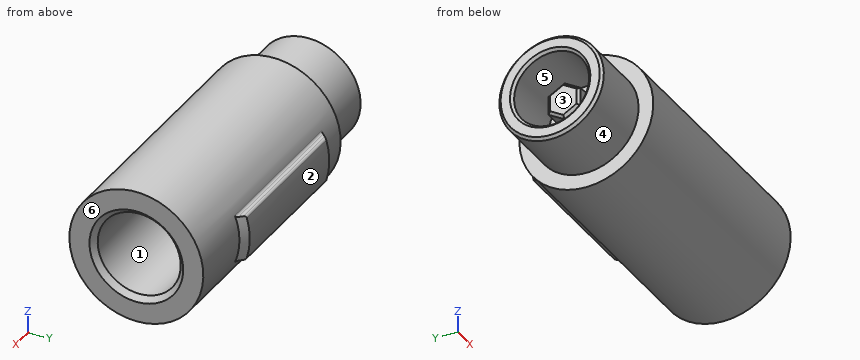
```python
from build123d import *

# Parameters (mm, degrees)
SKETCH_1_R          = 5
EXTRUDE_1_DEPTH     = 19
SKETCH_3_R          = 3.1
CUT_EXTRUDE_1_DEPTH = 17
EXTRUDE_2_DEPTH     = 12
SKETCH_8_R          = 3.9
EXTRUDE_4_DEPTH     = 5
SKETCH_9_R          = 2.8
CUT_EXTRUDE_2_DEPTH = 5
EXTRUDE_5_DEPTH     = 3.2
FILLET_1_R          = 0.2
CHAMFER_1_SIZE      = 0.5
CHAMFER_2_SIZE      = 0.4
CHAMFER_3_SIZE      = 0.2


with BuildPart() as part:
    # 草图1 → 凸台-拉伸1 (new body)
    with BuildSketch(Plane(origin=(0, 0, 0), x_dir=(0, 0, -1), z_dir=(1, 0, 0))):
        Circle(SKETCH_1_R)
    extrude(amount=EXTRUDE_1_DEPTH)

    # 草图3 → 切除-拉伸1 (cut)
    with BuildSketch(Plane(origin=(19, 0, 0), x_dir=(0, 0, -1), z_dir=(1, 0, 0))):
        Circle(SKETCH_3_R)
    extrude(amount=-CUT_EXTRUDE_1_DEPTH, mode=Mode.SUBTRACT)

    # 草图5 → 凸台-拉伸2 (add)
    with BuildSketch(Plane(origin=(2, 0, 0), x_dir=(0, 0, -1), z_dir=(1, 0, 0))):
        with BuildLine():
            Line((-1.688194302, 2.6), (1.688194302, 2.6))
            Line((1.688194302, 2.6), (1.688194302, 5.234500931))
            ThreePointArc((1.688194302, 5.234500931), (0, 5.5), (-1.688194302, 5.234500931))
            Line((-1.688194302, 5.234500931), (-1.688194302, 2.6))
        make_face()
    extrude(amount=EXTRUDE_2_DEPTH)

    # 草图8 → 凸台-拉伸4 (add)
    with BuildSketch(Plane.ZY):
        Circle(SKETCH_8_R)
    extrude(amount=EXTRUDE_4_DEPTH)

    # 草图9 → 切除-拉伸2 (cut)
    with BuildSketch(Plane.ZY.offset(5)):
        Circle(SKETCH_9_R)
    extrude(amount=-CUT_EXTRUDE_2_DEPTH, mode=Mode.SUBTRACT)

    # 草图10 → 凸台-拉伸5 (add)
    with BuildSketch(Plane.ZY):
        Polygon((0.692820323, 1.2), (-0.692820323, 1.2), (-1.385640646, 0), (-0.692820323, -1.2), (0.692820323, -1.2), (1.385640646, 0), align=None)
    extrude(amount=EXTRUDE_5_DEPTH)

    # 圆角1
    fillet_1_edges = [part.edges().sort_by_distance(p)[0] for p in [
        (8, 4.70637865, 1.688194302),
        (8, 5.234500931, 1.688194302),
        (8, 4.70637865, -1.688194302),
        (8, 5.234500931, -1.688194302),
    ]]
    fillet(fillet_1_edges, radius=FILLET_1_R)

    # 倒角1
    # the kernel refuses this chamfer: 0.5 mm, written as the material it takes off along each edge
    with BuildSketch(Plane(origin=(14, 0, 0), x_dir=(0, 0.8686030413593419, -0.4955085837211114), z_dir=(0, -0.4955085837211114, -0.8686030413593419))) as chamfer_1_piece_1:
        Polygon((5.5, -CHAMFER_1_SIZE), (5.5 - CHAMFER_1_SIZE, 0), (5.5, 0), align=None)
    revolve(axis=Axis((14, 0, 0), (1, 0, 0)), revolution_arc=59.40658503, mode=Mode.SUBTRACT)
    with BuildSketch(Plane(origin=(2, 0, 0), x_dir=(0, 0.8686030413593415, -0.4955085837211117), z_dir=(0, -0.4955085837211117, -0.8686030413593415))) as chamfer_1_piece_2:
        Polygon((5.5 - CHAMFER_1_SIZE, 0), (5.5, CHAMFER_1_SIZE), (5.5, 0), align=None)
    revolve(axis=Axis((2, 0, 0), (1, 0, 0)), revolution_arc=59.40658503, mode=Mode.SUBTRACT)
    with BuildSketch(Plane(origin=(14, 2.6, 2.974035796), x_dir=(0.027495876610585623, 0.9996219169112968, 0), z_dir=(0, 0, -1))) as chamfer_1_piece_3_section:
        Polygon((CHAMFER_1_SIZE * 0.999621916911, -CHAMFER_1_SIZE * 0.0274958766106), (-CHAMFER_1_SIZE * 0.0274958766106, -CHAMFER_1_SIZE * 0.999621916911), (0, 0), align=None)
    chamfer_1_piece_3 = extrude(amount=5.948071591, mode=Mode.PRIVATE)
    chamfer_1_piece_3 = chamfer_1_piece_3 & Plane(origin=(13.821912141, 0, 0), x_dir=(0, 0, -1), z_dir=(1, 0, 0)) * Cylinder(3.1, 14, mode=Mode.PRIVATE)
    add(chamfer_1_piece_3, mode=Mode.SUBTRACT)

    # 倒角2
    chamfer_2_edges = [part.edges().sort_by_distance(p)[0] for p in [
        (19, 0, 3.1),
    ]]
    chamfer(chamfer_2_edges, length=CHAMFER_2_SIZE)

    # 倒角3
    chamfer_3_edges = [part.edges().sort_by_distance(p)[0] for p in [
        (-5, 0, -3.9),
        (-5, 0, -2.8),
        (-3.2, 0.6, 1.039230485),
        (-3.2, 1.2, 0),
        (-3.2, 0.6, -1.039230485),
        (-3.2, -0.6, -1.039230485),
        (-3.2, -1.2, 0),
        (-3.2, -0.6, 1.039230485),
    ]]
    chamfer(chamfer_3_edges, length=CHAMFER_3_SIZE)


solid = part.part
```
Read the model definition and answer for the solid it produces. Units are mm, in the model's axes. Face numbers are marked on the shaded views. A direction names the side the tool comes from. Give positions to 0.01 mm unless a question says otherwise; leave off trailing zeros. Write each loop counter-clockwise with the first axis right and the second up, starting at its lowest first coordinate (ties: lowest second). Pieces come first, ordered by that corner, then holes. Notation, with made-up numbers: (-37, -33) - (3, -33) arc R19 ccw to (3, 2) - close; hole circle Ø11 at (53, 21.25). An arc over 180 degrees is marked (long way). Write item = value, one per line. Start each with the question number.
Item 1: Each of these flat-tipped pins is pushed along its axis until it touches: P1, Ø1, axis at x = 6.5, y = 2, coming from the +Z side; P2, Ø0.7, axis at x = -2, z = 0, coming from the +Y side; P3, Ø3, axis at y = 1, z = 0, coming from the -X side. Where does it stop, or does it pass through?
Item 2: Find the intervals of material crossed by probe 1 along Y at (x, z) = (-1.5, 0); probe 2 along Y at (x, z) = (13.25, 0); probe 3 along Y at (x, z) = (15.25, 0), in increasing order. Write a range as [from, to].
Item 3: Find section C-C (x = 10). Give the vertices of the cut face in (y, z), then the cut area to 3 significant figures.
Item 4: A tool of negligible diameter and unlimited length cuts with its end or side. For the marked faces 1, 2 and 3, from which of +Z, -Z, +X, -X, +Y, -Y can it reach the whole face along a straight path? Write none if from no direction.
Item 5: Find section A-A (x = -0.75). Give the vertices of the cut face in (y, z), then the cut area to 3 significant figures.
Item 6: The mould has two halves that part along Z. Classify the marked faces 4, 5 and 6: +Z half, -Z half, draft (parallel to the pull), parting line (faces both ways), or undercut.
Response:
q1.P1 = 4.77
q1.P2 = 3.9
q1.P3 = -3.2
q2.probe_1 = [-3.9, -2.8], [-1.2, 1.2], [2.8, 3.9]
q2.probe_2 = [-5, -3.1], [2.6, 5.5]
q2.probe_3 = [-5, -3.1], [3.1, 5]
q3.outline = (4.66, -1.82) arc R0.2 cw to (4.85, -1.69) - (5.09, -1.69) arc R0.2 ccw to (5.28, -1.54) arc R5.5 ccw to (5.28, 1.54) arc R0.2 ccw to (5.09, 1.69) - (4.85, 1.69) arc R0.2 cw to (4.66, 1.82) arc R5 ccw (long way) to start; hole (2.6, -1.69) - (2.6, 1.69) arc R3.1 ccw (long way) to start
q3.area = 51.2 mm²
q4.face_1 = +X
q4.face_2 = +X, -X, +Y
q4.face_3 = -X
q5.outline = circle Ø7.8 at (0, 0); (-1.2, -0.69) - (0, -1.39) - (1.2, -0.69) - (1.2, 0.69) - (0, 1.39) - (-1.2, 0.69) - close; hole circle Ø5.6 at (0, 0)
q5.area = 28.1 mm²
q6.face_4 = parting line
q6.face_5 = undercut
q6.face_6 = draft
